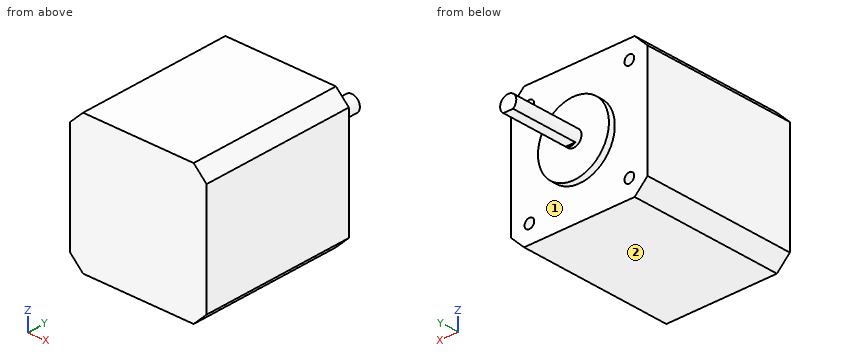
Autodesk Inventor part; units mm, degrees
ref_plane "YZ Plane" through (0, 0, 0) normal (1, 0, 0) x (0, 1, 0)
ref_plane "XZ Plane" through (0, 0, 0) normal (0, 1, 0) x (-1, 0, 0)
ref_plane "XY Plane" through (0, 0, 0) normal (0, 0, 1) x (1, 0, 0)
sketch "Sketch1" plane through (0, 0, 0) normal (0, 1, 0) x (-1, 0, 0)
  line L0 (0, 0) -> (42.3, 0)
  line L1 (42.3, 0) -> (42.3, 42.3)
  line L2 (42.3, 42.3) -> (0, 42.3)
  line L3 (0, 42.3) -> (0, 0)
  dimension "d0" = 42.3
  dimension "d1" = 42.3
extrude "Extrusion1" add sketch "Sketch1" along normal blind 48
sketch "Sketch2" plane through (0, 48, 0) normal (0, 1, 0) x (1, 0, 0)
  line L0 (0, 0) -> (-42.3, 0)
  line L1 (0, -42.3) -> (0, 0)
  circle A0 centre (-21.15, -21.15) radius 11
  point P0 (0, -2)
  point P1 (-2, 0)
  point P2 (-40.3, 0)
  point P3 (0, -40.3)
  dimension "d6" = 22
  dimension "d7" = 21.15
  dimension "d8" = 21.15
extrude "Extrusion2" add sketch "Sketch2" along normal blind 2
sketch "Sketch3" plane through (-21.15, 50, 21.15) normal (0, 1, 0) x (1, 0, 0)
  circle A0 centre (0, 0) radius 11
  circle A1 centre (0, 0) radius 2.5
  point P0 (21.15, 21.15)
  dimension "d11" = 5
extrude "Extrusion3" add sketch "Sketch3" along normal blind 22 contours A1
sketch "Sketch4" plane through (-21.15, 72, 21.15) normal (0, 1, 0) x (1, 0, 0)
  circle A0 centre (0, 0) radius 2.5
  line L0 (-1.5, 2) -> (1.5, 2)
  point P0 (21.15, 21.15)
  dimension "d14" = 2
extrude "Extrusion4" cut sketch "Sketch4" against normal blind 21 contours L0 A0 picked at (-0.3466, 2.0912)
sketch "Sketch5" plane through (0, 48, 0) normal (0, 1, 0) x (1, 0, 0)
  line L0 (-42.3, 0) -> (-42.3, -42.3)
  line L1 (-42.3, -42.3) -> (0, -42.3)
  circle A0 centre (-36.65, -5.65) radius 1.5
  circle A1 centre (-5.65, -5.65) radius 1.5
  circle A2 centre (-5.65, -36.65) radius 1.5
  circle A3 centre (-36.65, -36.65) radius 1.5
  point P0 (-42.3, -2)
  point P1 (-42.3, -40.3)
  point P2 (-40.3, -42.3)
  point P3 (-2, -42.3)
  point P4 (0, 0)
  dimension "d17" = 3
  dimension "d18" = 3
  dimension "d19" = 3
  dimension "d20" = 3
  dimension "d21" = 31
  dimension "d22" = 5.65
  dimension "d23" = 31
  dimension "d24" = 5.65
extrude "Extrusion5" cut sketch "Sketch5" against normal blind 4.5
chamfer "Chamfer1" distance 4 angle 45 4 edges at (-42.3, 24, 0) (-42.3, 24, 42.3) (0, 24, 0) (0, 24, 42.3)
properties part number "StepperMotorNema17x48mm"
Check sheet for the modelled part. Datum: model origin and axes. Units: mm. Face numbers are marked on the shaded views. A direction names the side the tool comes from. Give positions to 0.01 mm unless a question says otherwise; leave off trailing zeros. Loops run counter-clockwise (first coordinate to the right, second up) from the corner with the lowest first, then second, coordinate; pieces in that order, holes last. Notation, with made-up numbers: M -26.75,81 L 10.25,81 A31 ccw 10.25,106 Z; hole C 34,-1 d7. An arc over 180 degrees is marked long. Return JSON: item names as keys, results as strings. Group by question number.
1. Thickness scan on L1, parallel to X at y = 46.45, z = 36.65; L2, parallel to Z at x = -5.65, y = 44.75; L3, parallel to X at y = 44, z = 5. Record the ranges inside material, lowest first.
2. Cross-section at B-B on x = -21.15. Record the boundary of the cut face in (y, z), plus the area to 3 significant figures.
3. Cross-section at D-D on y = 47. Record the boundary of the cut face in (x, z), plus the area to 3 significant figures.
4. Cross-section at C-C on z = 5.65. Record the boundary of the cut face in (x, y), plus the area to 3 significant figures.
5. Go/stop test with flat-tipped pins: pin 1 (6.5 mm diameter, centred on x = -18, z = 16, fed in from +Y); pin 2 (3.5 mm diameter, centred on x = -5.5, z = 36, fed in from +Y); pin 3 (2.5 mm diameter, centred on x = -5.65, z = 36.65, fed in from +Y). Record where each tip stops, or that it passes through.
6. Cross-section at A-A on y = 29.5. Record the boundary of the cut face in (x, z), plus the area to 3 significant figures.
7. Tool access check on the marked faces 1 and 2. Record the directions out of +Z, -Z, +X, -X, +Y, -Y that give a thin tool (end or side, any length) a straight path to the whole face; none if there is none.
Return value:
{
 "1": {"L1": "-42.3 to -38.15, -35.15 to -7.15, -4.15 to 0", "L2": "0 to 4.15, 7.15 to 35.15, 38.15 to 42.3", "L3": "-42.3 to -38, -35.3 to -7, -4.3 to 0"},
 "2": {"outline": "M 0,0 L 48,0 L 48,10.15 L 50,10.15 L 50,18.65 L 51,18.65 L 51,19.15 L 72,19.15 L 72,23.65 L 50,23.65 L 50,32.15 L 48,32.15 L 48,42.3 L 0,42.3 Z", "area": "2,170 mm^2"},
 "3": {"outline": "M -42.3,4 L -38.3,0 L -4,0 L 0,4 L 0,38.3 L -4,42.3 L -38.3,42.3 L -42.3,38.3 Z; hole C -36.65,5.65 d3; hole C -36.65,36.65 d3; hole C -5.65,5.65 d3; hole C -5.65,36.65 d3", "area": "1,730 mm^2"},
 "4": {"outline": "M -42.3,0 L 0,0 L 0,48 L -4.15,48 L -4.15,43.5 L -7.15,43.5 L -7.15,48 L -35.15,48 L -35.15,43.5 L -38.15,43.5 L -38.15,48 L -42.3,48 Z", "area": "2,000 mm^2"},
 "5": {"pin 1": "y = 50", "pin 2": "y = 48", "pin 3": "y = 43.5"},
 "6": {"outline": "M -42.3,4 L -38.3,0 L -4,0 L 0,4 L 0,38.3 L -4,42.3 L -38.3,42.3 L -42.3,38.3 Z", "area": "1,760 mm^2"},
 "7": {"face 1": "+Y", "face 2": "-Z, +X, -X, +Y, -Y"}
}
